The drawing under review shows one solid part. Ordinate dimensions are in mm from its lowest x, y, z. A direction names the side the tool comes from. Give positions to 0.01 mm unless a question says otherwise; leave off trailing zeros. Loops run counter-clockwise (first coordinate to the right, second up) from the corner with the lowest first, then second, coordinate; pieces in that order, holes last. Notation, with made-up numbers: M 11,28.5 L 36,28.5 A23 ccw 36,37.5 Z; hole C 68,-31 d8. An arc over 180 degrees is marked long. Write item = value, one per line. Start each with the question number.
1. We need section D-D on y = 52.5. Give the boundary of the cut face in (x, z) (3 decimals), then the cut area to 3 significant figures.
2. Draft analysis for pull direction Y (two halves, no side actions). For the marked faces 3, 4, 5 and 6, state which applies: pulls with the +Y half, pulls with the -Y half, needs draft (parallel to the pull), parting line crosses it, or undercut.
3. For pin 1 (1 mm diameter, centred on x = 33, z = 28.5, fed in from +Y) (3 decimals); pin 2 (5 mm diameter, centred on y = 39.5, z = 6, fed in from -X); pin 3 (6 mm diameter, centred on y = 33.5, z = 17.5, fed in from +X); pin 4 (3 mm diameter, centred on y = 8, z = 19.5, fed in from -X) (3 decimals), all flat-tipped, find the tip position at first contact; note any pin that passes through.
4. We need section B-B on z = 19.05. Give the boundary of the cut face in (x, y) (3 decimals).
5. We need section C-C on x = 19.05. Give the boundary of the cut face in (y, z) (3 decimals).
6. Wall thickness on line 1 along Y through (x, z) = (7, 18.5) (3 decimals); line 2 along Y through (x, z) = (29, 9.5) (3 decimals); line 3 along X through (y, z) = (27.5, 26.5): over which ranges is each line inside the solid? List them lowest first. Write a range as from..to.
7. We need section A-A on x = 26. Give the boundary of the cut face in (y, z) (3 decimals).
8. For the marked faces 1 and 2, list the 3-axis set-ups (+Z, -Z, +X, -X, +Y, -Y) from which the entire face can be reached by the end or side of a thin tool; tool diameter is ignored.
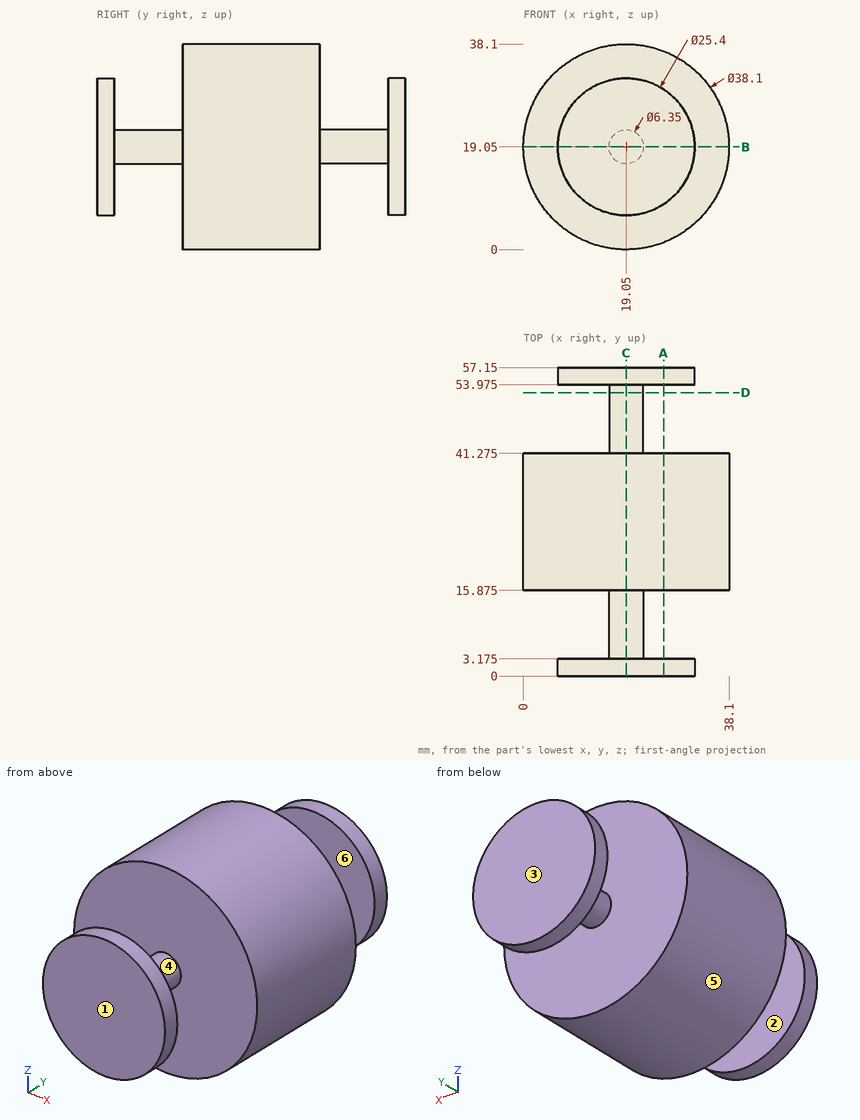
Final values:
q1.outline = C 19.05,19.05 d6.35
q1.area = 31.7 mm²
q2.face_3 = pulls with the +Y half
q2.face_4 = undercut
q2.face_5 = needs draft
q2.face_6 = undercut
q3.pin_1 = 41.275
q3.pin_2 = 3.19
q3.pin_3 = 38.1
q3.pin_4 = 15.875
q4.outline = M 0,15.875 L 15.875,15.875 L 15.875,3.175 L 6.35,3.175 L 6.35,0 L 31.75,0 L 31.75,3.175 L 22.225,3.175 L 22.225,15.875 L 38.1,15.875 L 38.1,41.275 L 22.225,41.275 L 22.225,53.975 L 31.75,53.975 L 31.75,57.15 L 6.35,57.15 L 6.35,53.975 L 15.875,53.975 L 15.875,41.275 L 0,41.275 Z
q5.outline = M 0,6.35 L 3.175,6.35 L 3.175,15.875 L 15.875,15.875 L 15.875,0 L 41.275,0 L 41.275,15.875 L 53.975,15.875 L 53.975,6.35 L 57.15,6.35 L 57.15,31.75 L 53.975,31.75 L 53.975,22.225 L 41.275,22.225 L 41.275,38.1 L 15.875,38.1 L 15.875,22.225 L 3.175,22.225 L 3.175,31.75 L 0,31.75 Z
q6.line_1 = 0..3.175, 15.875..41.275, 53.975..57.15
q6.line_2 = 15.875..41.275
q6.line_3 = 1.52..36.58
q7.outline = M 0,8.42 L 3.175,8.42 L 3.175,29.68 L 0,29.68 Z; M 15.875,1.313 L 41.275,1.313 L 41.275,36.787 L 15.875,36.787 Z; M 53.975,8.42 L 57.15,8.42 L 57.15,29.68 L 53.975,29.68 Z
q8.face_1 = +Z, -Z, +X, -X, -Y
q8.face_2 = none
